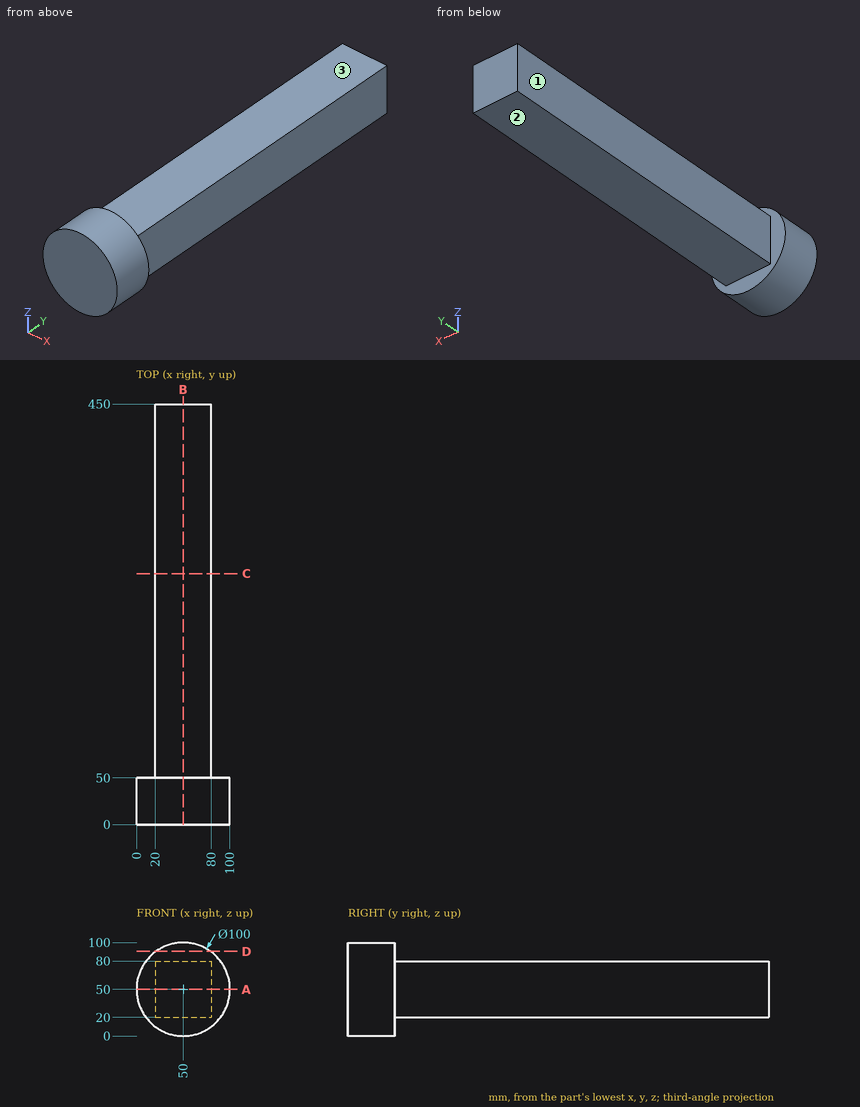
Study the drawing (mm; zero at the part's minimum x, y, z) and answer. A direction names the side the tool comes from. Give positions to 0.01 mm unless a question says otherwise; leave off trailing zeros. Loops run counter-clockwise (first coordinate to the right, second up) from the corner with the lowest first, then second, coordinate; pieces in that order, holes last. Notation, with made-up numbers: (6, 17.5) -> (34, 17.5) arc R16 cw to (34, 42.5) -> close; hole circle Ø1 at (-3, -5.5). An arc over 180 degrees is marked (long way). Write item = value, one per line. Start each with the question number.
(1) Find section D-D on z = 90.5. Give the vertices of the cut face in (x, y), and give its area (3 significant figures).
(2) Find the intervals of material crossed by probe 1 along Y at (x, z) = (92, 43.5); probe 2 along Z at (x, y) = (35.5, 286), in increasing order. Write a range as from..to.
(3) Find section C-C on y = 268.5. Give the vertices of the cut face in (x, z), and give its area (3 significant figures).
(4) Find section B-B on x = 50. Give the vertices of the cut face in (y, z).
(5) Which of the six approach directions +Z, -Z, +X, -X, +Y, -Y give full straight-line access (tool end or side, diameter ignored) to the marked faces 1, 2 and 3?
(6) Given pin 1 Ø3 at (x, y) = (40.5, 228) entering from -Z; pin 2 Ø6 at (y, z) = (256, 50) entering from -X; pin 3 Ø1 at (x, z) = (82.5, 67) entering from +Y, each flat-ended and moving along its own axis, determine where each tip first touches the part or whether it passes through.
(7) Find section A-A on z = 50. Give the vertices of the cut face in (x, y).
From the geometry:
q1.outline = (20.68, 0) -> (79.32, 0) -> (79.32, 50) -> (20.68, 50) -> close
q1.area = 2,930 mm^2
q2.probe_1 = 0..50
q2.probe_2 = 20..80
q3.outline = (20, 20) -> (80, 20) -> (80, 80) -> (20, 80) -> close
q3.area = 3,600 mm^2
q4.outline = (0, 0) -> (50, 0) -> (50, 20) -> (450, 20) -> (450, 80) -> (50, 80) -> (50, 100) -> (0, 100) -> close
q5.face_1 = +Z, -Z, -X, +Y
q5.face_2 = -Z, +X, -X, +Y
q5.face_3 = +Z, +X, -X, +Y
q6.pin_1 = 20
q6.pin_2 = 20
q6.pin_3 = 50
q7.outline = (0, 0) -> (100, 0) -> (100, 50) -> (80, 50) -> (80, 450) -> (20, 450) -> (20, 50) -> (0, 50) -> close
